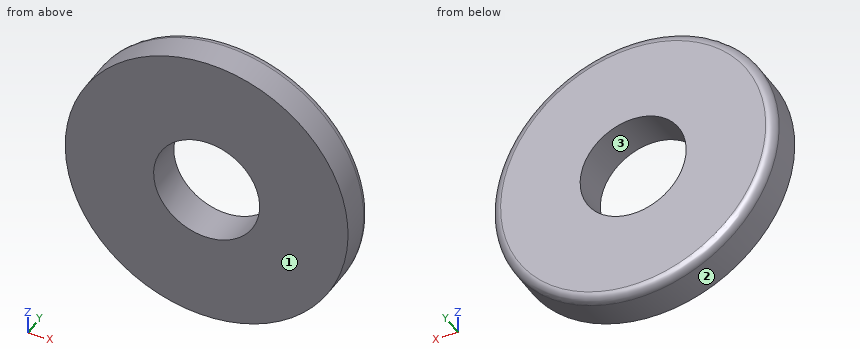
```python
from build123d import *

# Parameters (mm, degrees)
CROQUIS_BASE_R          = 4
SALIENTE_EXTRUIR3_DEPTH = 1.1
CROQUIS_BARRENO_R       = 1.5
CORTAR_EXTRUIR1_DEPTH   = 6.762811814
REDONDEO1_R             = 0.25


with BuildPart() as part:
    # Croquis base → Saliente-Extruir3 (new body)
    with BuildSketch(Plane(origin=(0, 0, 0), x_dir=(1, 0, 0), z_dir=(0, 1, 0))):
        with Locations(Location((0, 0, 0), (0, 0, 270))):
            Circle(CROQUIS_BASE_R)
    extrude(amount=SALIENTE_EXTRUIR3_DEPTH)

    # Croquis barreno → Cortar-Extruir1 (cut, through all)
    with BuildSketch(Plane(origin=(0, 1.1, 0), x_dir=(1, 0, 0), z_dir=(0, 1, 0))):
        with Locations(Location((0, 0, 0), (0, 0, 270))):
            Circle(CROQUIS_BARRENO_R)
    extrude(amount=-CORTAR_EXTRUIR1_DEPTH, mode=Mode.SUBTRACT)

    # Redondeo1
    redondeo1_edges = [part.edges().sort_by_distance(p)[0] for p in [
        (0, 1.1, -4),
    ]]
    fillet(redondeo1_edges, radius=REDONDEO1_R)


solid = part.part
```
The model under review builds one solid part; all positions refer to its coordinate system, in mm. Face numbers are marked on the shaded views. Round coordinates to 2 decimals unless told otherwise and drop trailing zeros. Write each loop counter-clockwise with the first axis right and the second up, starting at its lowest first coordinate (ties: lowest second). Pieces come first, ordered by that corner, then holes.
(1) Mouldability with a two-part tool opening along Z and no side actions: class the marked faces 1, 2 and 3 as +Z half, -Z half, draft (parallel to the pull), parting line (faces both ways), or undercut.
(2) Wall thickness on L1, parallel to X at y = 0.3, z = 0; L2, parallel to Z at x = -0.5, y = 0.5: over which ranges is each line inside the solid? List them lowest first.
(3) We need section B-B on z = 0. Give the boundary of the cut face in (x, y).
(4) We need section A-A on x = 0. Give the boundary of the cut face in (y, z), and give its area (3 significant figures).
Findings below:
1. face 1: draft
1. face 2: parting line
1. face 3: undercut
2. L1: x = -4 to -1.5, 1.5 to 4
2. L2: z = -3.97 to -1.41, 1.41 to 3.97
3. outline: (-4, 0) - (-1.5, 0) - (-1.5, 1.1) - (-3.75, 1.1) arc R0.25 ccw to (-4, 0.85) - close; (1.5, 0) - (4, 0) - (4, 0.85) arc R0.25 ccw to (3.75, 1.1) - (1.5, 1.1) - close
4. outline: (0, -4) - (0.85, -4) arc R0.25 ccw to (1.1, -3.75) - (1.1, -1.5) - (0, -1.5) - close; (0, 1.5) - (1.1, 1.5) - (1.1, 3.75) arc R0.25 ccw to (0.85, 4) - (0, 4) - close
4. area: 5.47 mm2
